Could you check a few things on this model? Use its own coordinates, in mm. A direction names the side the tool comes from. Coordinates: 2 decimals unless noted, no trailing zeros. Write each loop counter-clockwise with the first axis right and the second up, starting at its lowest first coordinate (ties: lowest second). Pieces come first, ordered by that corner, then holes.
Item 1: I want a section at A-A on x = 15. Please give me the cut outline in (y, z), then the cut area to 3 significant figures.
Item 2: If I drill on probe 1 along X at (y, z) = (15, 3.25); probe 2 along Y at (x, z) = (26, 14.75); probe 3 along Y at (x, z) = (15, 5.25), over which ranges is the centre line in solid material (lowest first)?
Item 3: I want a section at B-B on y = 90. Please give me the cut outline in (x, z), then the cut area to 3 significant figures.
Item 4: I want a section at D-D on x = 23.75. Please give me the cut outline in (y, z), then the cut area to 3 significant figures.
Item 5: Which directions (+Z, -Z, +X, -X, +Y, -Y) give clear straight access to the entire face, cutting with the end or side of a thin tool? Please do faces 4 (the cylindrical face through (1.43, 31, 10.14)), 5 (the flat face through (25, 4, 7)), 6 (the flat face through (15, 100, 10)), 7 (the flat face through (24, 32.5, 10)).
Item 6: For P1, Ø1, axis at y = 80, z = 17.5, coming from the -X side; P2, Ø2, axis at y = 63.5, z = 15.5, coming from the +X side; P3, Ø5, axis at x = 13.5, z = 9.5, coming from the -Y side; P4, Ø5.5, axis at x = 15, y = 15, coming from the +Z side, each with a flat end and sliding along its axis, tell me the tip position at first contact or that it passes through.
Item 7: Thinking about a two-plate mould opening in Y: for faces 1 (the cylindrical face through (28, 99, 10)), 2 (the flat face through (15, 51, 20)), 3 (the cylindrical face through (29, 82, 10)), which applies, +Y half, -Y half, draft (parallel to the pull), parting line (faces both ways), or undercut?
from build123d import *

# Parameters (mm, degrees)
F0_W      = 30
F0_H      = 100
F1_DEPTH  = 20
F2_R      = 12.5
F3_DEPTH  = 15
F4_R      = 3.5
F5_DEPTH  = 20
F6_R      = 3
F7_DEPTH  = 20
F8_W      = 7.5
F8_H      = 47.5
F9_DEPTH  = 20
F10_W     = 7.5
F10_H     = 47.5
F11_DEPTH = 20
F12_R     = 5
F13_R     = 5
F14_W     = 19.995708
F14_H     = 15
F15_DEPTH = 15


with BuildPart() as f1:
    # F0 (on Top) → F1 (new body)
    with BuildSketch(Plane.XY):
        with Locations((15, 50)):
            Rectangle(F0_W, F0_H)
    extrude(amount=F1_DEPTH)

    # F2 (on Top) → F3 (cut)
    with BuildSketch(Plane.XY):
        with Locations((15, 15)):
            Circle(F2_R)
    extrude(amount=F3_DEPTH, mode=Mode.SUBTRACT)

    # F4 (on Top) → F5 (cut)
    with BuildSketch(Plane.XY):
        with Locations((15, 15)):
            Circle(F4_R)
    extrude(amount=F5_DEPTH, mode=Mode.SUBTRACT)

    # F6 (on Top) → F7 (cut)
    with BuildSketch(Plane.XY):
        with Locations((15, 90)):
            Circle(F6_R)
    extrude(amount=F7_DEPTH, mode=Mode.SUBTRACT)

    # F8 (on Top) → F9 (cut)
    with BuildSketch(Plane.XY):
        with Locations((3.75, 56.25)):
            Rectangle(F8_W, F8_H)
    extrude(amount=F9_DEPTH, mode=Mode.SUBTRACT)

    # F10 (on Top) → F11 (cut)
    with BuildSketch(Plane.XY):
        with Locations((26.25, 56.25)):
            Rectangle(F10_W, F10_H)
    extrude(amount=F11_DEPTH, mode=Mode.SUBTRACT)

    # F12
    f12_edges = [f1.edges().sort_by_distance(p)[0] for p in [
        (30, 32.5, 10),
        (30, 0, 10),
        (0, 0, 10),
        (0, 32.5, 10),
    ]]
    fillet(f12_edges, radius=F12_R)

    # F13
    f13_edges = [f1.edges().sort_by_distance(p)[0] for p in [
        (0, 100, 10),
        (0, 80, 10),
        (30, 100, 10),
        (30, 80, 10),
    ]]
    fillet(f13_edges, radius=F13_R)

    # F14 (on Top) → F15 (cut)
    with BuildSketch(Plane.XY):
        with Locations((15.002146, 7.5)):
            Rectangle(F14_W, F14_H)
    extrude(amount=F15_DEPTH, mode=Mode.SUBTRACT)


solid = f1.part
Response values:
1. outline: (0, 15) - (11.5, 15) - (11.5, 20) - (0, 20) - close; (18.5, 15) - (27.5, 15) - (27.5, 0) - (87, 0) - (87, 20) - (18.5, 20) - close; (93, 0) - (100, 0) - (100, 20) - (93, 20) - close
1. area: 1,430 mm2
2. probe 1: x = 0 to 2.5, 27.5 to 30
2. probe 2: y = 0.1 to 9.06, 20.94 to 32.4, 80.1 to 99.9
2. probe 3: y = 27.5 to 87, 93 to 100
3. outline: (0, 0) - (12, 0) - (12, 20) - (0, 20) - close; (18, 0) - (30, 0) - (30, 20) - (18, 20) - close
3. area: 480 mm2
4. outline: (0, 15) - (23.93, 15) - (23.93, 0) - (32.5, 0) - (32.5, 20) - (0, 20) - close; (80, 0) - (100, 0) - (100, 20) - (80, 20) - close
4. area: 691 mm2
5. face 4: +Z, -Z, -X
5. face 5: -Z, -Y
5. face 6: +Z, -Z, +X, -X, +Y
5. face 7: +Z, -Z, +X
6. P1: stops at x = 2.82
6. P2: stops at x = 22.5
6. P3: stops at y = 26.84
6. P4: passes through
7. face 1: +Y half
7. face 2: draft
7. face 3: undercut
